```python
from build123d import *

# Parameters (mm, degrees)
SKETCH1_W           = 14.478
SKETCH1_H           = 1.27
BOSS_EXTRUDE1_DEPTH = 139.954
SKETCH2_W           = 14.478
SKETCH2_H           = 2.54
BOSS_EXTRUDE2_DEPTH = 3.683
LPATTERN1_COUNT     = 4
LPATTERN1_PITCH     = 30.48


with BuildPart() as part:
    # Sketch1 → Boss-Extrude1 (new body)
    with BuildSketch(Plane.XY):
        with Locations((7.239, 0.635)):
            Rectangle(SKETCH1_W, SKETCH1_H)
    extrude(amount=BOSS_EXTRUDE1_DEPTH)

    # Sketch2 → Boss-Extrude2 (add)
    with BuildSketch(Plane(origin=(0, 1.27, 0), x_dir=(1, 0, 0), z_dir=(0, 1, 0))):
        with Locations((7.239, -13.97)):
            Rectangle(SKETCH2_W, SKETCH2_H)
        with Locations((7.239, -34.29)):
            Rectangle(SKETCH2_W, SKETCH2_H)
    boss_extrude2 = extrude(amount=BOSS_EXTRUDE2_DEPTH)

    # LPattern1: Boss-Extrude2 ×4
    with Locations(*[(0, 0, i * LPATTERN1_PITCH) for i in range(1, LPATTERN1_COUNT)]):
        add(boss_extrude2)


solid = part.part
```
Geometry check sheet. Reference: the model listing, model coordinates, mm. A direction names the side the tool comes from. Coordinates: 2 decimals unless noted, no trailing zeros. Loops run counter-clockwise (first coordinate to the right, second up) from the corner with the lowest first, then second, coordinate; pieces in that order, holes last.
Item 1: Sectioned sample at B-B, the plane z = 87.5. Record the boundary of the cut face in (x, y), then the cut area to 3 significant figures.
Item 2: Access from +Z, -Z, +X, -X, +Y, -Y to the whole of each face (thin tool, end or side, straight path). Record for faces 1 (the face through (7, 1.27, 39)), 2 (the face through (7, 4.953, 14)), 3 (the face through (7, 3, 12.7)).
Item 3: Sectioned sample at A-A, the plane y = 2.95. Count the separate pieces of the cut face and the enclosed holes in it, then the cut area to 3 significant figures.
Item 4: Thickness scan on line 1 (Y direction, x = 9.25, z = 28.5). Record the ranges inside material, lowest first.
Item 5: Release check for a two-part mould opening along Z. For faces 4 (the face through (7, 3, 96.52)), 5 (the face through (7, 3, 127)), 6 (the face through (7, 4.953, 44)) record: released by +Z, released by -Z, zero draft, split by the parting line, or undercut.
Item 6: Go/stop test with flat-tipped pins: pin 1 Ø4.5 at (x, z) = (4, 54.5) entering from +Y; pin 2 Ø1.8 at (x, y) = (9.5, 3) entering from -Z; pin 3 Ø1.1 at (x, y) = (10, 2.5) entering from +Z. Record where each tip stops, or that it passes through.
Check result:
1. outline: (0, 0) - (14.48, 0) - (14.48, 1.27) - (0, 1.27) - close
1. area: 18.4 mm2
2. face 1: +X, -X, +Y
2. face 2: +Z, -Z, +X, -X, +Y
2. face 3: -Z, +X, -X, +Y
3. separate pieces: 8
3. enclosed holes: 0
3. area: 294 mm2
4. line 1: y = 0 to 1.27
5. face 4: undercut
5. face 5: released by +Z
5. face 6: zero draft
6. pin 1: stops at y = 1.27
6. pin 2: stops at z = 12.7
6. pin 3: stops at z = 127
